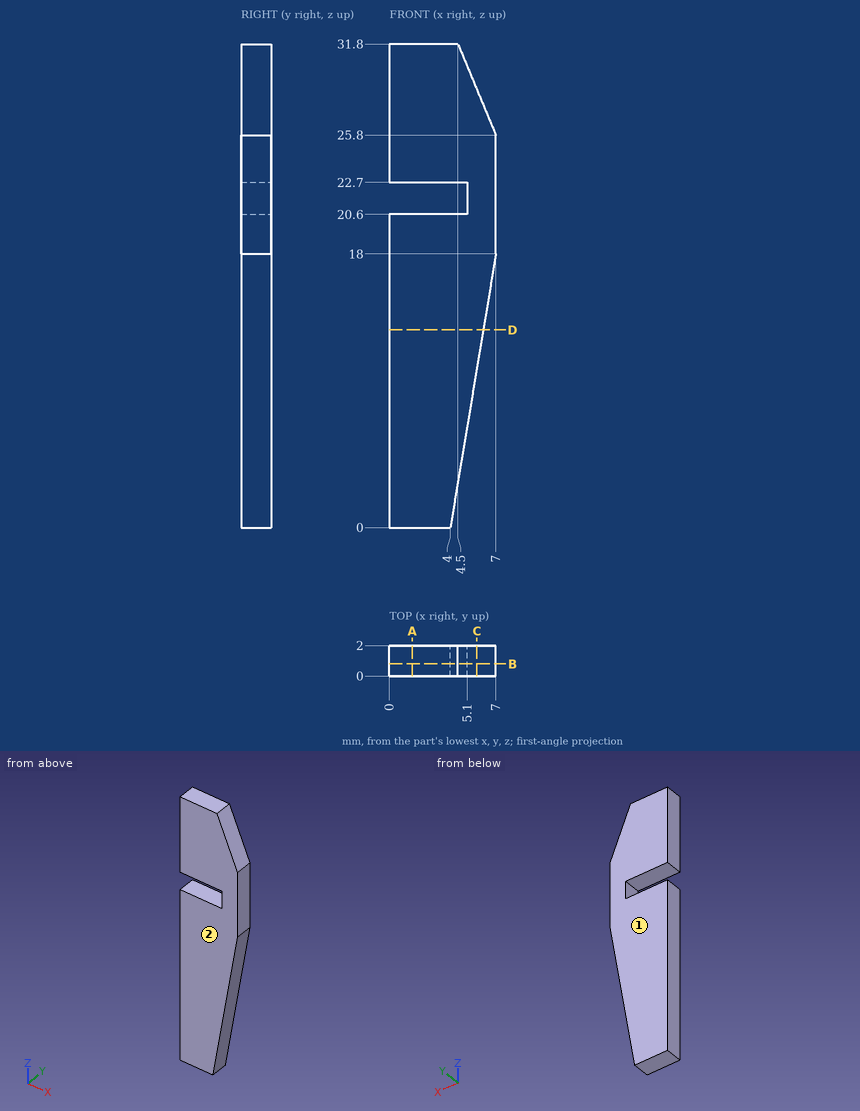
The figure shows three views and two pictorial views of one solid part (mm, origin at its lowest corner). Answer the questions. Round coordinates to 2 decimals unless told otherwise and drop trailing zeros. Order: outer loops, then holes, each group sorted by start corner. A loop starts at its lowest first (then second) coordinate and runs counter-clockwise, first axis right, second up. Notation, with made-up numbers: M 53,7 L 95,7 A26 ccw 95,37 Z; hole C -38.75,13.25 d9. An arc over 180 degrees is marked long. Put each result on its own line as item: value. Start each with the question number.
Q1. Section B-B, the plane y = 0.8 is taken. Write down the section's boundary in (x, z), and give its area (3 significant figures).
Q2. For a pull along Y with two mould halves and no side action, classify the marked faces 1 and 2 as pulls with the +Y half, pulls with the -Y half, needs draft (parallel to the pull), parting line crosses it, or undercut.
Q3. Straight lines are drawn through the part: L1, parallel to Z at x = 2.25, y = 1.55; L2, parallel to X at y = 1.95, z = 22; L3, parallel to X at y = 1.7, z = 29. For each, find the intervals that lie inside material, in ascending order. Write a range as [from, to].
Q4. Section C-C, the plane x = 5.75 is taken. Write down the section's boundary in (y, z), and give its area (3 significant figures).
Q5. Section D-D, the plane z = 13 is taken. Write down the section's boundary in (x, y), and give its area (3 significant figures).
Q6. Section A-A, the plane x = 1.5 is taken. Write down the section's boundary in (y, z), and give its area (3 significant figures).
Findings below:
1. outline: M 0,0 L 4,0 L 7,18 L 7,25.8 L 4.5,31.8 L 0,31.8 L 0,22.7 L 5.1,22.7 L 5.1,20.6 L 0,20.6 Z
1. area: 177 mm^2
2. face 1: pulls with the +Y half
2. face 2: pulls with the -Y half
3. L1: z = [0, 20.6], [22.7, 31.8]
3. L2: x = [5.1, 7]
3. L3: x = [0, 5.67]
4. outline: M 0,10.5 L 2,10.5 L 2,28.8 L 0,28.8 Z
4. area: 36.6 mm^2
5. outline: M 0,0 L 6.17,0 L 6.17,2 L 0,2 Z
5. area: 12.3 mm^2
6. outline: M 0,0 L 2,0 L 2,20.6 L 0,20.6 Z; M 0,22.7 L 2,22.7 L 2,31.8 L 0,31.8 Z
6. area: 59.4 mm^2
